Autodesk Inventor part; units mm, degrees
ref_plane "YZ Plane" through (0, 0, 0) normal (1, 0, 0) x (0, 1, 0)
ref_plane "XZ Plane" through (0, 0, 0) normal (0, 1, 0) x (-1, 0, 0)
ref_plane "XY Plane" through (0, 0, 0) normal (0, 0, 1) x (1, 0, 0)
sketch "Szkic1" plane through (0, 0, 0) normal (0, 1, 0) x (-1, 0, 0)
  circle A0 centre (0, 0) radius 75
  dimension "d0" = 150
extrude "Wyciągnięcie proste1" add sketch "Szkic1" along normal blind 6
sketch "Szkic2" plane through (0, 6, 0) normal (0, 1, 0) x (1, 0, 0)
  circle A0 centre (0, 0) radius 26
  dimension "d3" = 52
extrude "Wyciągnięcie proste2" cut sketch "Szkic2" against normal through all
sketch "Szkic4" plane through (0, 0, 0) normal (0, -1, 0) x (1, 0, 0)
  circle A0 centre (0, 0) radius 45
  circle A1 centre (0, 45) radius 3
  dimension "d10" = 90
  dimension "d11" = 6
extrude "Wyciągnięcie proste4" cut sketch "Szkic4" against normal blind 4 contours A1 A0 | A0 A1 picked at (-0.118, 43.9996) picked at (0.1052, 45.987)
sketch "Szkic5" plane through (0, 4, 45) normal (0, -1, 0) x (1, 0, 0)
  circle A0 centre (0, 0) radius 1.6
  point P0 (0, -45)
  dimension "d14" = 3.2
extrude "Wyciągnięcie proste5" cut sketch "Szkic5" against normal through all
pattern_circular "Szyk kołowy1" count 4 over 360 about axis through (0, 0, 0) along (0, 1, 0) of "Wyciągnięcie proste4", "Wyciągnięcie proste5"
sketch "Szkic6" plane through (0, 6, 0) normal (0, 1, 0) x (1, 0, 0)
  circle A0 centre (0, 0) radius 26
  circle A1 centre (0, 0) radius 32.5
  dimension "d20" = 65
extrude "Wyciągnięcie proste6" cut sketch "Szkic6" against normal blind 4
sketch "Szkic7" plane through (0, 6, 0) normal (0, 1, 0) x (1, 0, 0)
  circle A0 centre (0, 0) radius 37.5
  circle A1 centre (0, 0) radius 32.5
  dimension "d23" = 75
extrude "Wyciągnięcie proste7" add sketch "Szkic7" along normal blind 3
sketch "Szkic8" plane through (0, 6, 0) normal (0, 1, 0) x (1, 0, 0)
  circle A0 centre (0, 0) radius 75
  circle A1 centre (0, 0) radius 67.5
  dimension "d26" = 135
  dimension "d29" = 150
extrude "Wyciągnięcie proste8" add sketch "Szkic8" along normal blind 5
sketch "Szkic9" plane through (0, 11, 0) normal (0, 1, 0) x (1, 0, 0)
  circle A0 centre (0, 0) radius 67.5
  circle A1 centre (0, 0) radius 71.25
  circle A2 centre (0, 71.25) radius 1.65
  dimension "d30" = 142.5
  dimension "d31" = 3.3
extrude "Wyciągnięcie proste9" cut sketch "Szkic9" against normal through all contours A2 A1 | A1 A2 picked at (-0.0658, 70.7025) picked at (0.0634, 71.7949)
pattern_circular "Szyk kołowy2" count 6 over 360 about axis through (0, 0, 0) along (0, 1, 0) of "Wyciągnięcie proste9"
sketch "Szkic10" plane through (0, 0, 0) normal (0, -1, 0) x (1, 0, 0)
  circle A0 centre (0, -71.25) radius 1.65
  circle A1 centre (0, -71.25) radius 3
  point P0 (0, 0)
  dimension "d37" = 6
extrude "Wyciągnięcie proste10" cut sketch "Szkic10" against normal blind 4
pattern_circular "Szyk kołowy3" count 6 over 360 about axis through (0, 0, 0) along (0, 1, 0) of "Wyciągnięcie proste10"
properties part number "_Drukowanie 3D"
Work out the finished part from the listing and answer in its coordinate system (mm). A direction names the side the tool comes from. Give positions to 0.01 mm unless a question says otherwise; leave off trailing zeros. Loops run counter-clockwise (first coordinate to the right, second up) from the corner with the lowest first, then second, coordinate; pieces in that order, holes last. Notation, with made-up numbers: (25.5, -28) -> (69.5, -28) arc R28 ccw to (69.5, -9) -> close; hole circle Ø4 at (39.5, 70). An arc over 180 degrees is marked (long way). Put each result on its own line as item: value. Start each with the question number.
Item 1: The part is cut by section A-A (x = 18). Give the vertices of the cut face in (y, z).
Item 2: Each of these flat-tipped pins is pushed along its axis until it touches: P1, Ø5, axis at x = 30, z = 33, coming from the +Y side; P2, Ø3, axis at x = -62.5, z = -35.5, coming from the -Y side; P3, Ø5, axis at x = 37, y = 7, coming from the -Z side. Where does it stop, or does it pass through?
Item 3: Find the intervals of material crossed by L1, parallel to Z at x = 0, y = 4.75; L2, parallel to X at y = 5.3, z = 0; L3, parallel to Z at x = 4, y = 6.5, in increasing order. Write a range as [from, to].
Item 4: The mould has two halves that part along X. Classify faces 4 (the face through (1, 4, -73)), 5 (the face through (1, 0, -32)), 6 (the face through (0.36, 7.55, 69.64)): released by +X, released by -X, zero draft, split by the parting line, or undercut.
Item 5: Which of the six approach directions +Z, -Z, +X, -X, +Y, -Y give full straight-line access (tool end or side, diameter ignored) to faces 1 (the face through (-29, 6, -29)), 2 (the face through (-43.58, 4.99, 0.74)), 3 (the face through (43.7, 4, -1.3))?
Answers below:
1. outline: (0, -72.81) -> (11, -72.81) -> (11, -65.06) -> (6, -65.06) -> (6, -32.9) -> (9, -32.9) -> (9, -27.06) -> (2, -27.06) -> (2, -18.76) -> (0, -18.76) -> close; (0, 18.76) -> (2, 18.76) -> (2, 27.06) -> (9, 27.06) -> (9, 32.9) -> (6, 32.9) -> (6, 65.06) -> (11, 65.06) -> (11, 72.81) -> (0, 72.81) -> close
2. P1: y = 6
2. P2: y = 4
2. P3: z = -66.59
3. L1: [-75, -72.9], [-69.6, -46.6], [-43.4, -32.5], [32.5, 43.4], [46.6, 69.6], [72.9, 75]
3. L2: [-75, -46.6], [-43.4, -32.5], [32.5, 43.4], [46.6, 75]
3. L3: [-74.89, -67.38], [-37.29, -32.25], [32.25, 37.29], [67.38, 74.89]
4. face 4: undercut
4. face 5: zero draft
4. face 6: undercut
5. face 1: +Y
5. face 2: +Y, -Y
5. face 3: -Y
